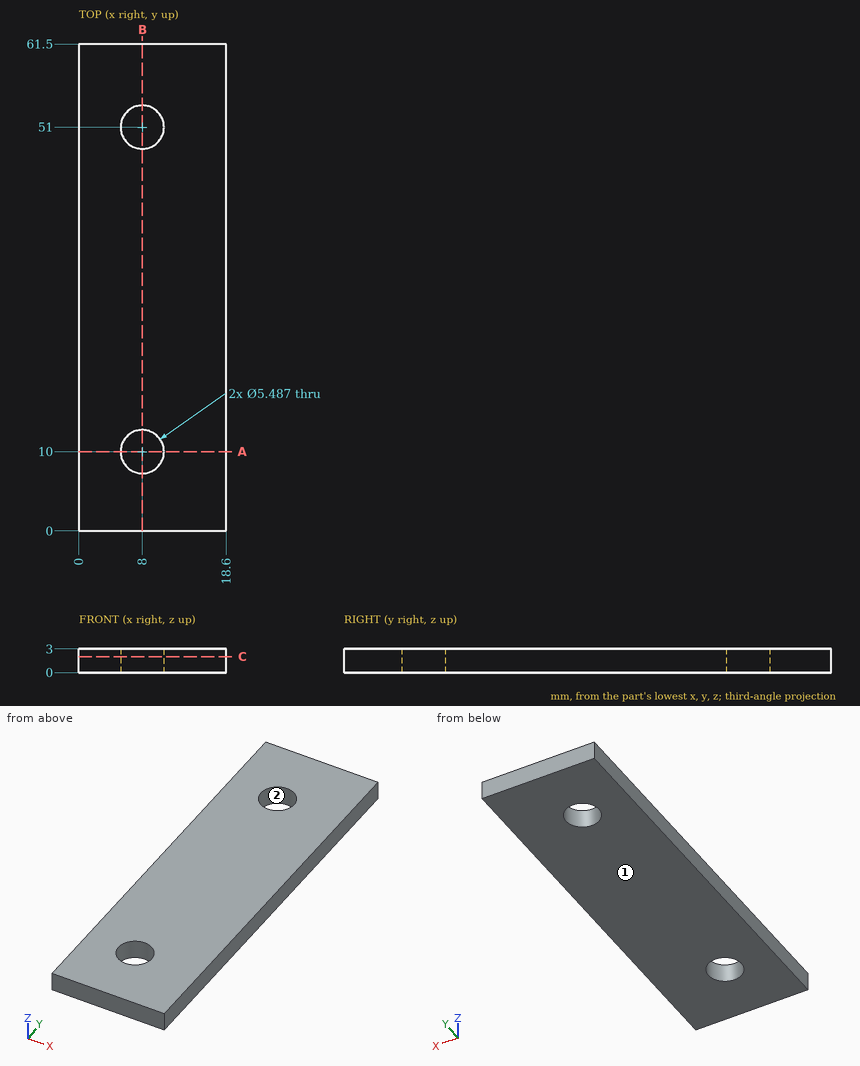
Geometry: see drawing. Coordinates: mm, zero at the bounding-box minimum. Round coordinates to 2 decimals unless told otherwise and drop trailing zeros. Write each loop counter-clockwise with the first axis right and the second up, starting at its lowest first coordinate (ties: lowest second). Pieces come first, ordered by that corner, then holes.
1) Cut plane C-C (z = 2). Return the cut outline in (x, y).
2) Draft query along Y for the marked faces 1 and 2. Return one class per face: pulls with the +Y half, pulls with the -Y half, needs draft (parallel to the pull), parting line crosses it, or undercut.
3) Cut plane A-A (y = 10). Return the cut outline in (x, z).
4) Contact query for flat-ended pins moving along their axis: P1, Ø1.5, axis at x = 6.5, y = 23.5, coming from the -Z side; P2, Ø5, axis at x = 8, y = 51, coming from the -Z side. Output: stop coordinate, or through.
5) Ray query, L1, parallel to Y at x = 8, z = 2.3; L2, parallel to Y at x = 6.75, z = 1.9; L3, parallel to X at y = 49.5, z = 1.7. Return the intervals inside material, ascending.
6) Cut plane B-B (x = 8). Return the cut outline in (y, z).
Geometry says:
1. outline: (0, 0) - (18.6, 0) - (18.6, 61.5) - (0, 61.5) - close; hole circle Ø5.49 at (8, 10); hole circle Ø5.49 at (8, 51)
2. face 1: needs draft
2. face 2: undercut
3. outline: (0, 0) - (5.26, 0) - (5.26, 3) - (0, 3) - close; (10.74, 0) - (18.6, 0) - (18.6, 3) - (10.74, 3) - close
4. P1: stops at z = 0
4. P2: passes through
5. L1: y = 0 to 7.26, 12.74 to 48.26, 53.74 to 61.5
5. L2: y = 0 to 7.56, 12.44 to 48.56, 53.44 to 61.5
5. L3: x = 0 to 5.7, 10.3 to 18.6
6. outline: (0, 0) - (7.26, 0) - (7.26, 3) - (0, 3) - close; (12.74, 0) - (48.26, 0) - (48.26, 3) - (12.74, 3) - close; (53.74, 0) - (61.5, 0) - (61.5, 3) - (53.74, 3) - close
